Input: part model. Units: mm. Frame: model coordinates. A direction names the side the tool comes from. Give positions to 0.01 mm unless a question says otherwise; leave off trailing zeros. Loops run counter-clockwise (first coordinate to the right, second up) from the corner with the lowest first, then second, coordinate; pieces in that order, holes last. Notation, with made-up numbers: (-21, 84.5) - (17, 84.5) arc R11 ccw to (17, 101.5) - close; hole circle Ø11 at (36, 7.25). An arc over 180 degrees is marked (long way). One line per item, written item: value.
from build123d import *

# Parameters (mm, degrees)
SKETCH_1_W      = 35.5
SKETCH_1_H      = 15
EXTRUDE_1_DEPTH = 19.25
SKETCH_2_W      = 35.5
SKETCH_2_H      = 15
SKETCH_2_W_2    = 6.6
SKETCH_2_R      = 2.1
EXTRUDE_2_DEPTH = 2
SKETCH_3_W      = 35.5
SKETCH_3_H      = 15
EXTRUDE_3_DEPTH = 7.25
SKETCH_4_R      = 3.649626988
EXTRUDE_4_DEPTH = 4.25


with BuildPart() as part:
    # 草图1 → 凸台-拉伸1 (new body)
    with BuildSketch(Plane(origin=(0, 0, 0), x_dir=(1, 0, 0), z_dir=(0, 1, 0))):
        with Locations((17.75, 7.5)):
            Rectangle(SKETCH_1_W, SKETCH_1_H)
    extrude(amount=EXTRUDE_1_DEPTH)

    # 草图2 → 凸台-拉伸2 (add)
    # profile 1 of 3: a face of its own
    with BuildSketch(Plane(origin=(0, 19.25, 0), x_dir=(1, 0, 0), z_dir=(0, 1, 0))):
        with Locations((17.75, 7.5)):
            Rectangle(SKETCH_2_W, SKETCH_2_H)
    # profile 2 of 3: a face of its own
    with BuildSketch(Plane(origin=(0, 19.25, 0), x_dir=(1, 0, 0), z_dir=(0, 1, 0))):
        with Locations((38.8, 7.5)):
            Rectangle(SKETCH_2_W_2, SKETCH_2_H)
        with Locations(Location((39.05, 3.75, 0), (0, 0, 270))):
            Circle(SKETCH_2_R, mode=Mode.SUBTRACT)
        with Locations(Location((39.05, 11.25, 0), (0, 0, 270))):
            Circle(SKETCH_2_R, mode=Mode.SUBTRACT)
    # profile 3 of 3: a face of its own
    with BuildSketch(Plane(origin=(0, 19.25, 0), x_dir=(1, 0, 0), z_dir=(0, 1, 0))):
        with Locations((-3.3, 7.5)):
            Rectangle(SKETCH_2_W_2, SKETCH_2_H)
        with Locations(Location((-3.55, 3.75, 0), (0, 0, 270))):
            Circle(SKETCH_2_R, mode=Mode.SUBTRACT)
        with Locations(Location((-3.55, 11.25, 0), (0, 0, 270))):
            Circle(SKETCH_2_R, mode=Mode.SUBTRACT)
    extrude(amount=EXTRUDE_2_DEPTH)

    # 草图3 → 凸台-拉伸3 (add)
    with BuildSketch(Plane(origin=(0, 21.25, 0), x_dir=(1, 0, 0), z_dir=(0, 1, 0))):
        with Locations((17.75, 7.5)):
            Rectangle(SKETCH_3_W, SKETCH_3_H)
    extrude(amount=EXTRUDE_3_DEPTH)

    # 草图4 → 凸台-拉伸4 (add)
    with BuildSketch(Plane(origin=(0, 28.5, 0), x_dir=(1, 0, 0), z_dir=(0, 1, 0))):
        with Locations(Location((28.3, 7.5, 0), (0, 0, 90))):
            Circle(SKETCH_4_R)
    extrude(amount=EXTRUDE_4_DEPTH)


solid = part.part
Item 1: Section A-A, the plane x = 39.05. Output: boundary loops of the cut face in (y, z), and give its area (3 significant figures).
Verdict:
outline: (19.25, -15) - (21.25, -15) - (21.25, -13.35) - (19.25, -13.35) - close; (19.25, -9.15) - (21.25, -9.15) - (21.25, -5.85) - (19.25, -5.85) - close; (19.25, -1.65) - (21.25, -1.65) - (21.25, 0) - (19.25, 0) - close
area: 13.2 mm^2
Item 2: Access query for faces 4 (the face through (27.2, 30.6, -10.98)), 5 (the face through (0, 9, -7)), 6 (the face through (35.5, 9, -7)), 7 (the face through (0, 25, -7)). Directions: +Z, -Z, +X, -X, +Y, -Y. A direction counts if a zero-diameter tool reaches every point of the face in a straight line with its end or side. Return the directions, or none.
Verdict:
face 4: +Y
face 5: +Z, -Z, -X, -Y
face 6: +Z, -Z, +X, -Y
face 7: +Z, -Z, -X, +Y
Item 3: Pin query (flat end, axial travel): P1, Ø2, axis at y = 24, z = -10, coming from the +X side; P2, Ø3.5, axis at x = -2, z = -6.5, coming from the +Y side; P3, Ø5.5, axis at x = -3.55, z = -3.75, coming from the -Y side. Return the tip coordinate at first contact, or that it passes through.
Verdict:
P1: stops at x = 35.5
P2: stops at y = 21.25
P3: stops at y = 19.25
Item 4: Material intervals for L1, parallel to X at y = 19.8, z = -11.25; L2, parallel to Z at x = -3, y = 20; L3, parallel to Y at x = 40, z = -6, sorted ascending.
Verdict:
L1: x = -6.6 to -5.65, -1.45 to 36.95, 41.15 to 42.1
L2: z = -15 to -13.28, -9.22 to -5.78, -1.72 to 0
L3: y = 19.25 to 21.25
Item 5: Section C-C, the plane x = 28.3. Output: boundary loops of the cut face in (y, z).
Verdict:
outline: (0, -15) - (28.5, -15) - (28.5, -11.15) - (32.75, -11.15) - (32.75, -3.85) - (28.5, -3.85) - (28.5, 0) - (0, 0) - close
Item 6: Section D-D, the plane z = -7.25. Output: boundary loops of the cut face in (x, y), and give its area (3 significant figures).
Verdict:
outline: (-6.6, 19.25) - (0, 19.25) - (0, 0) - (35.5, 0) - (35.5, 19.25) - (42.1, 19.25) - (42.1, 21.25) - (35.5, 21.25) - (35.5, 28.5) - (31.94, 28.5) - (31.94, 32.75) - (24.66, 32.75) - (24.66, 28.5) - (0, 28.5) - (0, 21.25) - (-6.6, 21.25) - close
area: 1,070 mm^2
Item 7: Section B-B, the plane z = -9.75. Output: boundary loops of the cut face in (x, y), and give its area (3 significant figures).
Verdict:
outline: (-6.6, 19.25) - (-5.02, 19.25) - (-5.02, 21.25) - (-6.6, 21.25) - close; (-2.08, 19.25) - (0, 19.25) - (0, 0) - (35.5, 0) - (35.5, 19.25) - (37.58, 19.25) - (37.58, 21.25) - (35.5, 21.25) - (35.5, 28.5) - (31.17, 28.5) - (31.17, 32.75) - (25.43, 32.75) - (25.43, 28.5) - (0, 28.5) - (0, 21.25) - (-2.08, 21.25) - close; (40.52, 19.25) - (42.1, 19.25) - (42.1, 21.25) - (40.52, 21.25) - close
area: 1,050 mm^2
Item 8: Draft query along Z for faces 1 (the face through (-3.46, 20.24, -13.35)), 2 (the face through (42.1, 20, -7)), 3 (the face through (17, 14, -15)). Return one class per face: pulls with the +Z half, pulls with the -Z half, needs draft (parallel to the pull), parting line crosses it, or undercut.
Verdict:
face 1: undercut
face 2: needs draft
face 3: pulls with the -Z half
